The model under review builds one solid part; all positions refer to its coordinate system, in mm. Face numbers are marked on the shaded views. A direction names the side the tool comes from. Give positions to 0.01 mm unless a question says otherwise; leave off trailing zeros. Write each loop counter-clockwise with the first axis right and the second up, starting at its lowest first coordinate (ties: lowest second). Pieces come first, ordered by that corner, then holes. Notation, with made-up numbers: (30, 67) - (73, 67) arc R22 ccw to (73, 77) - close; hole circle Ø10 at (-33, 38.25). An arc over 180 degrees is marked (long way). Write item = value, one per line.
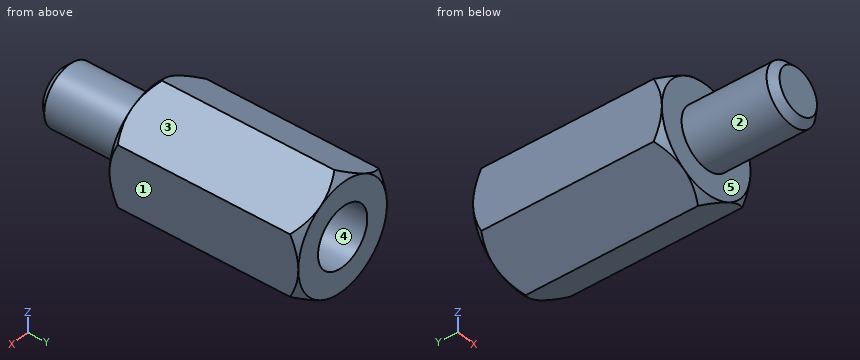
```python
from build123d import *

# Parameters (mm, degrees)
SKETCH1_R           = 1.25
BOSS_EXTRUDE1_DEPTH = 3.9
BOSS_EXTRUDE2_DEPTH = 8
SKETCH3_R           = 1.25
CUT_EXTRUDE1_DEPTH  = 4.8
SKETCH4_OUTSIDE_W   = 35.048
SKETCH4_OUTSIDE_H   = 35.744
SKETCH4_OUTSIDE_R   = 2.25
CUT_EXTRUDE2_DEPTH  = 12.9
CUT_EXTRUDE2_TAPER  = 45
SKETCH5_OUTSIDE_W   = 27.248
SKETCH5_OUTSIDE_H   = 27.944
SKETCH5_OUTSIDE_R   = 2.25
CUT_EXTRUDE3_DEPTH  = 9
CUT_EXTRUDE3_TAPER  = 45
CHAMFER1_SIZE       = 0.3


with BuildPart() as part:
    # Sketch1 → Boss-Extrude1 (new body)
    with BuildSketch(Plane(origin=(0, 0, 0), x_dir=(1, 0, 0), z_dir=(0, 1, 0))):
        Circle(SKETCH1_R)
    extrude(amount=BOSS_EXTRUDE1_DEPTH)

    # Sketch2 → Boss-Extrude2 (add)
    with BuildSketch(Plane(origin=(0, 3.9, 0), x_dir=(1, 0, 0), z_dir=(0, 1, 0))):
        Polygon((0, -2.598076211), (2.25, -1.299038106), (2.25, 1.299038106), (0, 2.598076211), (-2.25, 1.299038106), (-2.25, -1.299038106), align=None)
    extrude(amount=BOSS_EXTRUDE2_DEPTH)

    # Sketch3 → Cut-Extrude1 (cut)
    with BuildSketch(Plane(origin=(0, 11.9, 0), x_dir=(1, 0, 0), z_dir=(0, 1, 0))):
        Circle(SKETCH3_R)
    extrude(amount=-CUT_EXTRUDE1_DEPTH, mode=Mode.SUBTRACT)

    # Sketch4 outside → Cut-Extrude2 (cut, through all)
    with BuildSketch(Plane(origin=(0, 11.9, 0), x_dir=(1, 0, 0), z_dir=(0, 1, 0))):
        Rectangle(SKETCH4_OUTSIDE_W, SKETCH4_OUTSIDE_H)
        Circle(SKETCH4_OUTSIDE_R, mode=Mode.SUBTRACT)
    extrude(amount=-CUT_EXTRUDE2_DEPTH, taper=CUT_EXTRUDE2_TAPER, mode=Mode.SUBTRACT)

    # Sketch5 outside → Cut-Extrude3 (cut, through all)
    with BuildSketch(Plane.XZ.offset(-3.9)):
        Rectangle(SKETCH5_OUTSIDE_W, SKETCH5_OUTSIDE_H)
        Circle(SKETCH5_OUTSIDE_R, mode=Mode.SUBTRACT)
    extrude(amount=-CUT_EXTRUDE3_DEPTH, taper=CUT_EXTRUDE3_TAPER, mode=Mode.SUBTRACT)

    # Chamfer1
    chamfer1_edges = [part.edges().sort_by_distance(p)[0] for p in [
        (-1.25, 0, 0),
    ]]
    chamfer(chamfer1_edges, length=CHAMFER1_SIZE)


solid = part.part
```
1. Insertion check: P1, Ø2, axis at x = -1.5, z = 1, coming from the -Y side; P2, Ø2, axis at x = 0.5, y = 8, coming from the -Z side; P3, Ø0.8, axis at x = 0.5, z = 0.5, coming from the +Y side. Each pin has a flat end and moves straight along its axis. Give the tip position at first contact, or say it passes through.
Findings below:
P1 = 0
P2 = -2.6
P3 = 7.1
2. Machinability: for the marked faces 1 and 2, which of the approach directions +Z, -Z, +X, -X, +Y, -Y give a long, thin tool a straight path to every point of the face, cutting with its end or side? Answer none if there is none.
Findings below:
face_1 = +Z, -Z, +X, +Y, -Y
face_2 = -Y
3. Draft analysis for pull direction X (two halves, no side actions). For the marked faces 3, 4 and 5, state which applies: +X half, -X half, draft (parallel to the pull), parting line (faces both ways), or undercut.
Findings below:
face_3 = +X half
face_4 = undercut
face_5 = draft
4. Take a section at C-C on y = 3.25. Give the boundary of the cut face in (x, z), and give its area (3 significant figures).
Findings below:
outline = circle Ø2.5 at (0, 0)
area = 4.91 mm²
5. Take a section at B-B on y = 5. Give the boundary of the cut face in (x, z), and give its area (3 significant figures).
Findings below:
outline = (-2.25, -1.3) - (0, -2.6) - (2.25, -1.3) - (2.25, 1.3) - (0, 2.6) - (-2.25, 1.3) - close
area = 17.5 mm²
6. Take a section at A-A on y = 10.25. Give the boundary of the cut face in (x, z), and give its area (3 significant figures).
Findings below:
outline = (-2.25, -1.3) - (0, -2.6) - (2.25, -1.3) - (2.25, 1.3) - (0, 2.6) - (-2.25, 1.3) - close; hole circle Ø2.5 at (0, 0)
area = 12.6 mm²
7. For line 1 (X direction, y = 9.1, z = 0); line 2 (Y direction, x = -0.2, z = 1.95); line 3 (X direction, y = 10.5, z = -0.7), list the stretches that pass through material, from the lowest coordinate up. Write a range as from..to.
Findings below:
line_1 = -2.25..-1.25, 1.25..2.25
line_2 = 3.9..11.9
line_3 = -2.25..-1.04, 1.04..2.25
